Verification items for this drawing (mm, ordinates from the low corner). Round coordinates to 2 decimals unless told otherwise and drop trailing zeros. Write each loop counter-clockwise with the first axis right and the second up, starting at its lowest first coordinate (ties: lowest second). Pieces come first, ordered by that corner, then holes. Notation, with made-up numbers: (57, -29.75) -> (99, -29.75) arc R20 ccw to (99, 5.25) -> close; hole circle Ø1 at (80, 61). An arc over 180 degrees is marked (long way). Put each result on its own line as item: value. Start each with the question number.
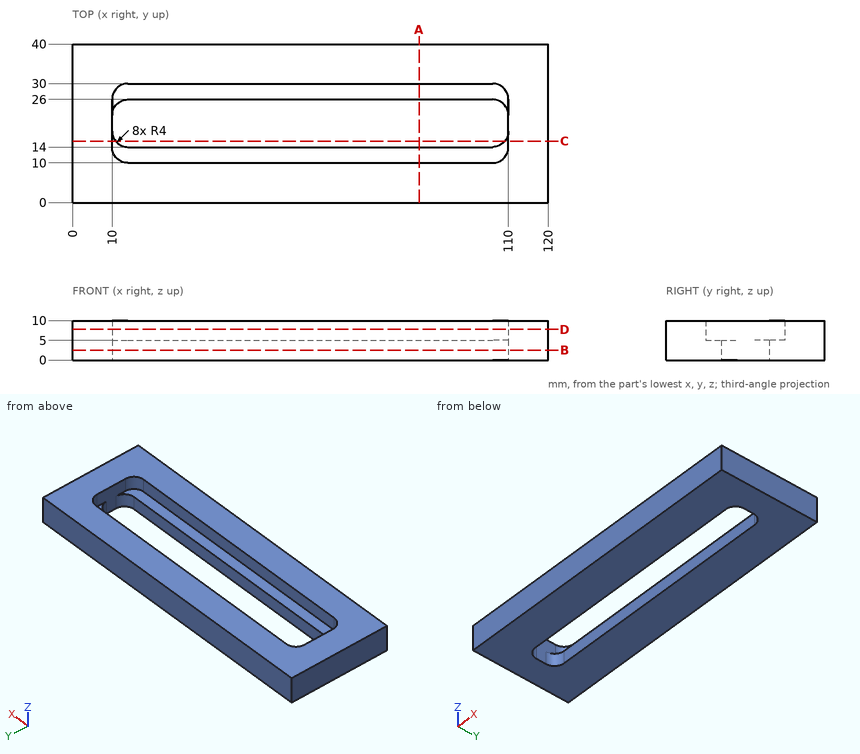
1. Section check C-C, the plane y = 15.5. Enter the section's corners in (x, z), then the cut area to 3 significant figures.
2. Gauge pin test, flat end, axial feed: P1, Ø2.5, axis at x = 61.5, y = 26, coming from the +Z side. Record the tip position at first contact, or that the pin passes through.
3. Section check D-D, the plane z = 7.75. Enter the section's corners in (x, y).
4. Section check B-B, the plane z = 2.5. Enter the section's corners in (x, y).
5. Section check A-A, the plane x = 87.5. Enter the section's corners in (y, z), then the cut area to 3 significant figures.
6. Material ranges on L1, parallel to Y at x = 36.5, z = 1.75; L2, parallel to Y at x = 77.5, z = 8; L3, parallel to X at y = 14.5, z = 9.75, recorded low to high. Write a range as [from, to].
Reply:
1. outline: (0, 0) -> (10.88, 0) -> (10.88, 5) -> (10, 5) -> (10, 10) -> (0, 10) -> close; (109.12, 0) -> (120, 0) -> (120, 10) -> (110, 10) -> (110, 5) -> (109.12, 5) -> close
1. area: 209 mm2
2. P1: stops at z = 5
3. outline: (0, 0) -> (120, 0) -> (120, 40) -> (0, 40) -> close; hole (10, 14) arc R4 ccw to (14, 10) -> (106, 10) arc R4 ccw to (110, 14) -> (110, 26) arc R4 ccw to (106, 30) -> (14, 30) arc R4 ccw to (10, 26) -> close
4. outline: (0, 0) -> (120, 0) -> (120, 40) -> (0, 40) -> close; hole (10, 18) arc R4 ccw to (14, 14) -> (106, 14) arc R4 ccw to (110, 18) -> (110, 22) arc R4 ccw to (106, 26) -> (14, 26) arc R4 ccw to (10, 22) -> close
5. outline: (0, 0) -> (14, 0) -> (14, 5) -> (10, 5) -> (10, 10) -> (0, 10) -> close; (26, 0) -> (40, 0) -> (40, 10) -> (30, 10) -> (30, 5) -> (26, 5) -> close
5. area: 240 mm2
6. L1: y = [0, 14], [26, 40]
6. L2: y = [0, 10], [30, 40]
6. L3: x = [0, 10], [110, 120]
